Read the model definition and answer for the solid it produces. Units are mm, in the model's axes. Round coordinates to 2 decimals unless told otherwise and drop trailing zeros. Loops run counter-clockwise (first coordinate to the right, second up) from the corner with the lowest first, then second, coordinate; pieces in that order, holes last. Notation, with made-up numbers: M 50,-18 L 67,-18 A10 ccw 67,-2 Z; hole C -17.75,68 d5. An arc over 180 degrees is marked long. Write each question's results on one line, items separated by ' | '.
from build123d import *

# Parameters (mm, degrees)
SKETCH_1_W                = 146
SKETCH_1_H                = 10
EXTRUDE_146X10_DEPTH      = 3
F_12MM_START              = 3
SKETCH_2_R                = 3
F_12MM_DEPTH              = 12
M2P5_DEPTH                = 75.692703794
M2P5_DEPTH_BACK           = 75.692703794
SKETCH_3_R                = 1.4
CUT_EXTRUDE_M3_DEPTH      = 75.692703794
CUT_EXTRUDE_M3_DEPTH_BACK = 75.692703794
SKETCH_4_W                = 3.4
SKETCH_4_H                = 5.4


with BuildPart() as part:
    # 草图1 → 主板轻量横条146x10 (new body)
    with BuildSketch(Plane.XY):
        Rectangle(SKETCH_1_W, SKETCH_1_H)
    extrude(amount=EXTRUDE_146X10_DEPTH)

    # 草图2 → 主板12mm支柱 (add)
    with BuildSketch(Plane.XY.offset(F_12MM_START)):
        with Locations((-24.5, 0)):
            Circle(SKETCH_2_R)
        with Locations((24.5, 0)):
            Circle(SKETCH_2_R)
    extrude(amount=F_12MM_DEPTH)

    # 草图3 → 主板M2p5通孔 (cut, two sides: drawn at the far end of the back side and taken through both)
    with BuildSketch(Plane.XY.offset(-M2P5_DEPTH_BACK)):
        with Locations((-24.5, 0)):
            Circle(SKETCH_3_R)
        with Locations((24.5, 0)):
            Circle(SKETCH_3_R)
    extrude(amount=M2P5_DEPTH + M2P5_DEPTH_BACK, mode=Mode.SUBTRACT)

    # 草图4 → 梁上M3调节槽 (cut, two sides: drawn at the far end of the back side and taken through both)
    with BuildSketch(Plane.XY.offset(-CUT_EXTRUDE_M3_DEPTH_BACK)):
        with Locations((-66.6, 0)):
            Rectangle(SKETCH_4_W, SKETCH_4_H)
        with Locations((66.6, 0)):
            Rectangle(SKETCH_4_W, SKETCH_4_H)
    extrude(amount=CUT_EXTRUDE_M3_DEPTH + CUT_EXTRUDE_M3_DEPTH_BACK, mode=Mode.SUBTRACT)


solid = part.part
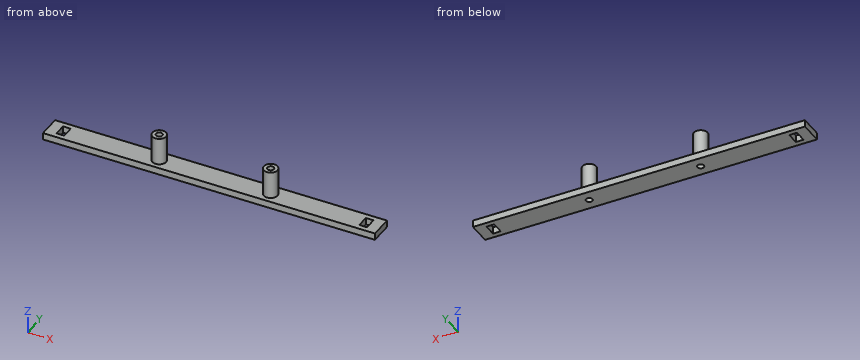
Item 1: The part is cut by section B-B (x = 24.5). Determine the outline of the cut face in (y, z).
Outcome:
outline: M -5,0 L -1.4,0 L -1.4,15 L -3,15 L -3,3 L -5,3 Z; M 1.4,0 L 5,0 L 5,3 L 3,3 L 3,15 L 1.4,15 Z
Item 2: Straight lines are drawn through the part: line 1 (Y direction, x = -24.5, z = 12); line 2 (X direction, y = 1.25, z = 7); line 3 (X direction, y = -1, z = 2.25). For each, find the intervals that lie inside material, in ascending order.
Outcome:
line 1: y = -3 to -1.4, 1.4 to 3 | line 2: x = -27.23 to -25.13, -23.87 to -21.77, 21.77 to 23.87, 25.13 to 27.23 | line 3: x = -73 to -68.3, -64.9 to -25.48, -23.52 to 23.52, 25.48 to 64.9, 68.3 to 73
Item 3: The part is cut by section C-C (z = 8.5). Determine the outline of the cut face in (x, y).
Outcome:
outline: C -24.5,0 d6; C 24.5,0 d6; hole C -24.5,0 d2.8; hole C 24.5,0 d2.8
Item 4: A flat-ended cylindrical pin translates along its axis: pin 1 (1.5 mm diameter, centred on y = 0, z = 8, fed in from +X). Find the tip coordinate at first contact, or state that the pin passes through.
Outcome:
pin 1: stops at x = 27.5
Item 5: The part is cut by section A-A (y = 0). Determine the outline of the cut face in (x, z).
Outcome:
outline: M -73,0 L -68.3,0 L -68.3,3 L -73,3 Z; M -64.9,0 L -25.9,0 L -25.9,15 L -27.5,15 L -27.5,3 L -64.9,3 Z; M -23.1,0 L 23.1,0 L 23.1,15 L 21.5,15 L 21.5,3 L -21.5,3 L -21.5,15 L -23.1,15 Z; M 25.9,0 L 64.9,0 L 64.9,3 L 27.5,3 L 27.5,15 L 25.9,15 Z; M 68.3,0 L 73,0 L 73,3 L 68.3,3 Z
